Check sheet for the drawn part. Datum: minimum x, y, z corner. Units: mm. A direction names the side the tool comes from. Give positions to 0.01 mm unless a question says otherwise; leave off trailing zeros. Loops run counter-clockwise (first coordinate to the right, second up) from the corner with the lowest first, then second, coordinate; pieces in that order, holes last.
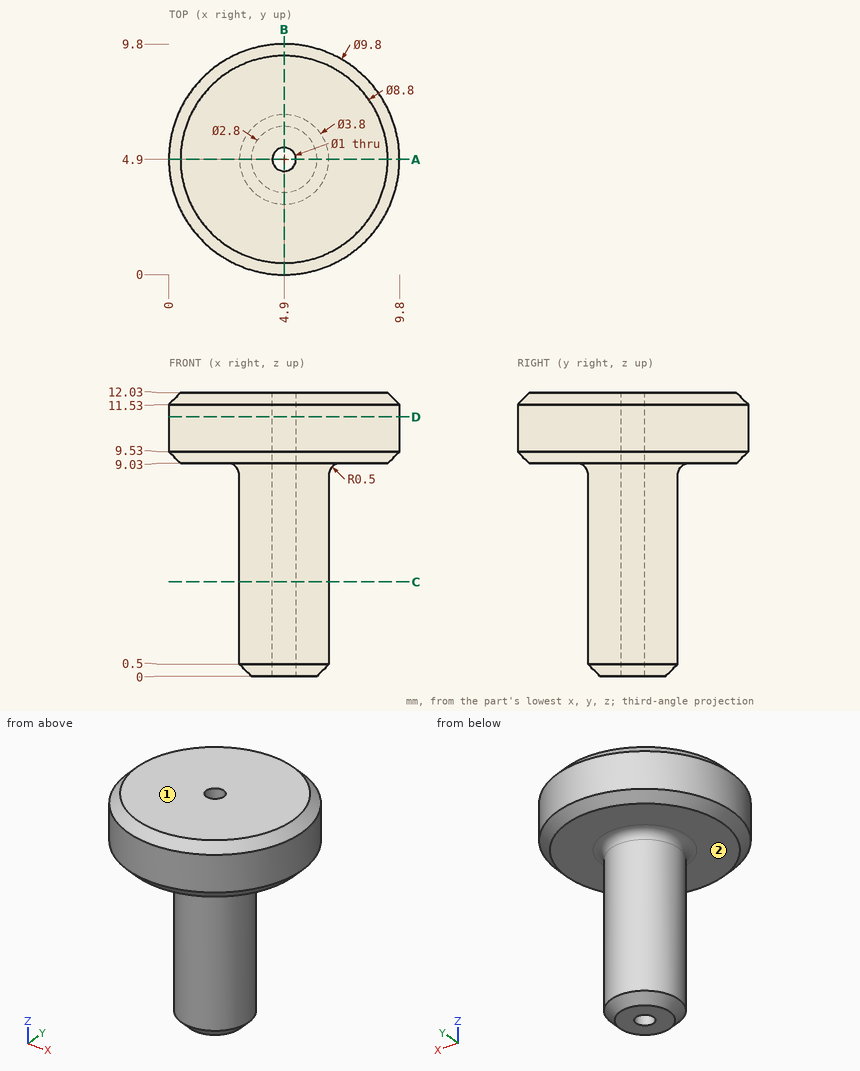
(1) Section check D-D on z = 11. Record the boundary of the cut face in (x, y), plus the area to 3 significant figures.
(2) Gauge pin test, flat ends, axial feed: pin 1 Ø1 at (y, z) = (8, 10.5) entering from -X; pin 2 Ø4 at (y, z) = (8.5, 1.5) entering from -X. Record the tip position at first contact, or that the pin passes through.
(3) Material ranges on line 1 (Z direction, x = 7.5, y = 1.5); line 2 (Y direction, x = 4.9, z = 2.5); line 3 (Y direction, x = 4.9, z = 9.25), recorded low to high.
(4) Section check C-C on z = 4. Record the boundary of the cut face in (x, y).
(5) Access from +Z, -Z, +X, -X, +Y, -Y to the whole of each face (thin tool, end or side, straight path). Record for the marked faces 1 and 2.
(6) Section check A-A on y = 4.9. Record the boundary of the cut face in (x, z).
Computed values:
1. outline: circle Ø9.8 at (4.9, 4.9); hole circle Ø1 at (4.9, 4.9)
1. area: 74.6 mm2
2. pin 1: stops at x = 0.75
2. pin 2: stops at x = 3.88
3. line 1: z = 9.03 to 12.03
3. line 2: y = 3 to 4.4, 5.4 to 6.8
3. line 3: y = 0.28 to 4.4, 5.4 to 9.52
4. outline: circle Ø3.8 at (4.9, 4.9); hole circle Ø1 at (4.9, 4.9)
5. face 1: +Z, +X, -X, +Y, -Y
5. face 2: -Z
6. outline: (0, 9.53) - (0.5, 9.03) - (2.5, 9.03) arc R0.5 cw to (3, 8.53) - (3, 0.5) - (3.5, 0) - (4.4, 0) - (4.4, 12.03) - (0.5, 12.03) - (0, 11.53) - close; (5.4, 0) - (6.3, 0) - (6.8, 0.5) - (6.8, 8.53) arc R0.5 cw to (7.3, 9.03) - (9.3, 9.03) - (9.8, 9.53) - (9.8, 11.53) - (9.3, 12.03) - (5.4, 12.03) - close
